Drawing for the job (mm, zero at the part's lowest x, y, z). Give positions to 0.01 mm unless a question says otherwise; leave off trailing zeros. Loops run counter-clockwise (first coordinate to the right, second up) from the corner with the lowest first, then second, coordinate; pieces in that order, holes last. Notation, with made-up numbers: M 11,44.25 L 44,44.25 A31 cw 44,81.25 Z; hole C 54,-26.5 d3. An arc over 180 degrees is marked long. Use CSV: the item, a comma, the result in double quotes. Start each with the question number.
(1) Wall check: line 1 along Y through (x, z) = (2, 4) (3 decimals); line 2 along X through (y, z) = (76, 3.75); line 3 along X through (y, z) = (89, 2.5). Give the ranges that are in metal, low to high. Write a range as from..to.
(2) Flat gauge pin, fed straight in: P1, Ø1, axis at y = 59.5, z = 5.5, coming from the +X side. Where does the tip first touch, or does it go through?
(3) Slice it at B-B on x = 6. List the corners of the cut face in (y, z) (3 decimals), and give its area (3 significant figures).
(4) Slice it at A-A on z = 4. List the corners of the cut face in (x, y) (3 decimals), and give its area (3 significant figures).
(5) Slice it at C-C on y = 136. List the corners of the cut face in (x, z), and give its area (3 significant figures).
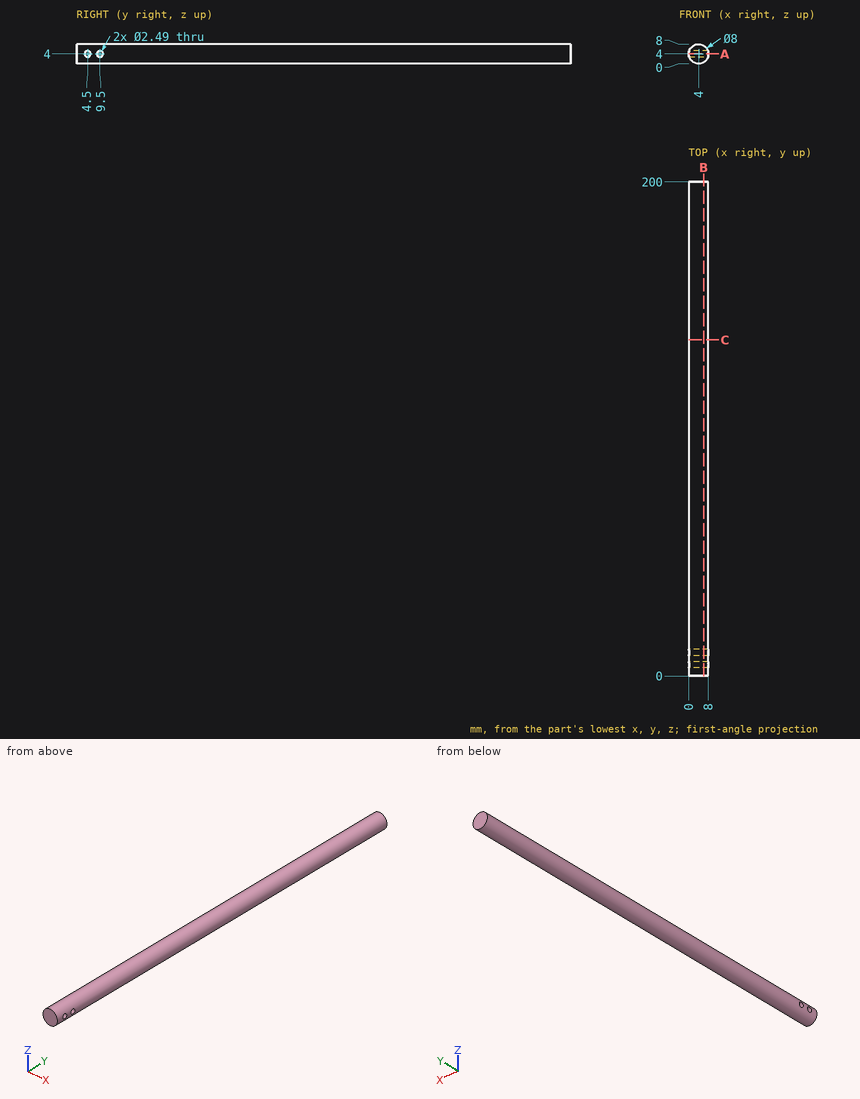
Reply:
1,line 1,"y = 0..3.255, 5.745..8.255, 10.745..200"
1,line 2,"x = 0.01..7.99"
1,line 3,"x = 0.29..7.71"
2,P1,"stops at x = 7.87"
3,outline,"M 0,0.536 L 200,0.536 L 200,7.464 L 0,7.464 Z; hole C 4.5,4 d2.49; hole C 9.5,4 d2.49"
3,area,"1,380 mm^2"
4,outline,"M 0,0 L 8,0 L 8,3.255 L 0,3.255 Z; M 0,5.745 L 8,5.745 L 8,8.255 L 0,8.255 Z; M 0,10.745 L 8,10.745 L 8,200 L 0,200 Z"
4,area,"1,560 mm^2"
5,outline,"C 4,4 d8"
5,area,"50.3 mm^2"
